CAD build for the part. Positions are in the model's coordinates, mm. A direction names the side the tool comes from. Round coordinates to 2 decimals unless told otherwise and drop trailing zeros. Loops run counter-clockwise (first coordinate to the right, second up) from the corner with the lowest first, then second, coordinate; pieces in that order, holes last.
from build123d import *

# Parameters (mm, degrees)
F0_W     = 152.4
F0_H     = 38.1
F1_DEPTH = 12.7
F2_SIZE2 = 10.16
F2_SIZE  = 25.4
F3_SIZE2 = 10.16
F3_SIZE  = 76.2
F4_W     = 11.8357492981
F4_H     = 10.9219625592
F5_DEPTH = 25.4


with BuildPart() as f1:
    # F0 (on Right) → F1 (new body, symmetric)
    with BuildSketch(Plane.YZ):
        with Locations((-38.1, 12.7)):
            Rectangle(F0_W, F0_H)
    extrude(amount=F1_DEPTH, both=True)

    # F2
    f2_edges = [f1.edges().sort_by_distance(p)[0] for p in [
        (12.7, -114.3, 12.7),
    ]]
    f2_side = f1.faces().sort_by_distance((12.7, -38.1, 12.7))[0]
    chamfer(f2_edges, length=F2_SIZE, length2=F2_SIZE2, reference=f2_side)

    # F3
    f3_edges = [f1.edges().sort_by_distance(p)[0] for p in [
        (12.7, 38.1, 12.7),
    ]]
    f3_side = f1.faces().sort_by_distance((12.7, -25.4, 12.7))[0]
    chamfer(f3_edges, length=F3_SIZE, length2=F3_SIZE2, reference=f3_side)

    # F4 (on face) → F5 (cut)
    with BuildSketch(Plane.XY.offset(31.75)):
        with Locations((-6.7821253509, -75.2695389092)):
            Rectangle(F4_W, F4_H)
    extrude(amount=-F5_DEPTH, mode=Mode.SUBTRACT)


solid = f1.part
Item 1: Cut at C-C (y = -9.5). List the corners of the cut face in (x, z).
Verdict:
outline: (-12.7, -6.35) - (8.89, -6.35) - (8.89, 31.75) - (-12.7, 31.75) - close
Item 2: Flat gauge pins, fed straight in: P1, Ø8, axis at y = 2.5, z = 15.5, coming from the +X side; P2, Ø3.5, axis at x = -4.5, y = -74.5, coming from the +Z side; P3, Ø5.5, axis at y = -73.5, z = 20.5, coming from the -X side. Where does each tip first touch, or does it go through?
Verdict:
P1: stops at x = 7.82
P2: stops at z = 6.35
P3: stops at x = -0.86
Item 3: Cut at A-A (z = 2.5). List the corners of the cut face in (x, y).
Verdict:
outline: (-12.7, -114.3) - (2.54, -114.3) - (12.7, -88.9) - (12.7, -38.1) - (2.54, 38.1) - (-12.7, 38.1) - close
Item 4: Cut at D-D (z = 13). List the corners of the cut face in (x, y).
Verdict:
outline: (-12.7, -114.3) - (2.54, -114.3) - (12.7, -88.9) - (12.7, -38.1) - (2.54, 38.1) - (-12.7, 38.1) - (-12.7, -69.81) - (-0.86, -69.81) - (-0.86, -80.73) - (-12.7, -80.73) - close
Item 5: Cut at B-B (x = -7). List the corners of the cut face in (y, z), plus the area to 3 significant figures.
Verdict:
outline: (-114.3, -6.35) - (38.1, -6.35) - (38.1, 31.75) - (-69.81, 31.75) - (-69.81, 6.35) - (-80.73, 6.35) - (-80.73, 31.75) - (-114.3, 31.75) - close
area: 5,530 mm2
Item 6: 3-axis set-ups, long thin cutter, end or side, ignore diameter. For faces 1 (the flat face through (-7, -69.809, 19)), 2 (the flat face through (0, -39, 31.75)): which of +Z, -Z, +X, -X, +Y, -Y reach the whole face in a straight line?
Verdict:
face 1: +Z, -X
face 2: +Z, +X, -X, +Y, -Y
Item 7: Mould opens along Y. For faces 3 (the flat face through (-0.864, -75, 19)), 4 (the flat face through (7.55, 0.53, 12.43)), 5 (the flat face through (12.7, -64, 13)) say: released by +Y, released by -Y, zero draft, split by the parting line, or undercut.
Verdict:
face 3: undercut
face 4: released by +Y
face 5: zero draft
Item 8: Wall check: L1, parallel to Y at x = -3.75, z = 15; L2, parallel to X at y = 11.5, z = 10; L3, parallel to X at y = -38, z = 22.5. Give the ranges that are in metal, low to high.
Verdict:
L1: y = -114.3 to -80.73, -69.81 to 38.1
L2: x = -12.7 to 6.09
L3: x = -12.7 to 12.69
